Work out the finished part from the listing and answer in its coordinate system (mm). A direction names the side the tool comes from. Coordinates: 2 decimals unless noted, no trailing zeros. Order: outer loops, then holes, each group sorted by start corner. A loop starts at its lowest first (then second) coordinate and runs counter-clockwise, first axis right, second up. Notation, with made-up numbers: (57, 15) - (89, 15) arc R31 ccw to (89, 42) - close; hole circle Ø4 at (26, 23). An arc over 180 degrees is marked (long way). Answer as a JSON object with one key per item and string values. Group by question number.
1) A tool of negligible diameter and unlimited length cuts with its end or side. For faces 5 (the face through (-0.867, 3.905, -0.035)), 6 (the face through (0, -5, 2.5)), 7 (the face through (0, -5, -2.5)), from which of +Z, -Z, +X, -X, +Y, -Y can it reach the whole face along a straight path? Write none if from no direction.
2) Find the intervals of material crossed by line 1 along Y through (x, z) = (0, -3.1); line 2 along Z through (x, y) = (14, -11.5); line 3 along Y through (x, z) = (0, -0.3), in increasing order.
3) The mould has two halves that part along X. Classify faces 1 (the face through (10, -21, -3.5)), 2 (the face through (-20.633, -15.821, -0.204)), 3 (the face through (-2.994, -22.804, 2.746)), 4 (the face through (-2.994, 22.804, -2.993)): released by +X, released by -X, zero draft, split by the parting line, or undercut.
4) Section C-C (y = 13.5) is taken. Give the vertices of the cut face in (x, z).
5) Section D-D (z = 0.5) is taken. Give the vertices of the cut face in (x, y).
6) Section A-A (x = 0) is taken. Give the vertices of the cut face in (y, z).
7) Each of these flat-tipped pins is pushed along its axis until it touches: P1, Ø1, axis at x = -12.5, z = 0.5, coming from the +Y side; P2, Ø2, axis at x = 18, y = -11.5, coming from the -Z side; P3, Ø1.5, axis at x = -18.5, z = -0.5, coming from the +Y side. Where does it stop, or does it pass through?
Autodesk Inventor part; units mm, degrees
ref_plane "YZ Plane" through (0, 0, 0) normal (1, 0, 0) x (0, 1, 0)
ref_plane "XZ Plane" through (0, 0, 0) normal (0, 1, 0) x (-1, 0, 0)
ref_plane "XY Plane" through (0, 0, 0) normal (0, 0, 1) x (1, 0, 0)
sketch "Sketch1" plane through (0, 0, 0) normal (0, 0, 1) x (1, 0, 0)
  circle A0 centre (0, 0) radius 23
  circle A1 centre (0, 0) radius 4
  dimension "d0" = 46
  dimension "d1" = 8
extrude "Extrusion1" add sketch "Sketch1" along normal mid plane 5
sketch "Sketch2" plane through (0, 0, 2.5) normal (0, 0, 1) x (1, 0, 0)
  circle A0 centre (0, 0) radius 23
  circle A1 centre (0, 0) radius 26
  dimension "d4" = 52
extrude "Extrusion2" add sketch "Sketch2" against normal blind 6 and the other way blind 0.5
properties part number "Rueda"
Report:
{
 "1": {"face 5": "+Z, -Z", "face 6": "+Z", "face 7": "-Z"},
 "2": {"line 1": "y = -26 to -23, 23 to 26", "line 2": "z = -2.5 to 2.5", "line 3": "y = -26 to -4, 4 to 26"},
 "3": {"face 1": "zero draft", "face 2": "split by the parting line", "face 3": "undercut", "face 4": "undercut"},
 "4": {"outline": "(-22.22, -3.5) - (-18.62, -3.5) - (-18.62, -2.5) - (18.62, -2.5) - (18.62, -3.5) - (22.22, -3.5) - (22.22, 3) - (18.62, 3) - (18.62, 2.5) - (-18.62, 2.5) - (-18.62, 3) - (-22.22, 3) - close"},
 "5": {"outline": "circle Ø52 at (0, 0); hole circle Ø8 at (0, 0)"},
 "6": {"outline": "(-26, -3.5) - (-23, -3.5) - (-23, -2.5) - (-4, -2.5) - (-4, 2.5) - (-23, 2.5) - (-23, 3) - (-26, 3) - close; (4, -2.5) - (23, -2.5) - (23, -3.5) - (26, -3.5) - (26, 3) - (23, 3) - (23, 2.5) - (4, 2.5) - close"},
 "7": {"P1": "stops at y = 23.07", "P2": "stops at z = -2.5", "P3": "stops at y = 19"}
}
